Geometry: final body of the model. Coordinates: model frame, mm. A direction names the side the tool comes from. Give positions to 0.01 mm unless a question says otherwise; leave off trailing zeros. Order: outer loops, then holes, each group sorted by start corner. A loop starts at its lowest first (then second) coordinate and runs counter-clockwise, first axis right, second up. Notation, with made-up numbers: (-1.75, 65) -> (4.25, 65) arc R17 cw to (4.25, 96) -> close; hole circle Ø7 at (64.25, -30). An arc over 180 degrees is marked (long way). One line per question, with ' | ' between items. Start each with the question number.
(1) Section D-D (z = 27). Return loops of the section in (x, y), then the cut area to 3 significant figures.
(2) Section C-C (x = -8). Return loops of the section in (y, z), then the cut area to 3 significant figures.
(3) Set-up query: faces 1 (the face through (-18, 0, 9)), 2 (the face through (-44.45, -5, 6)), 3 (the face through (-33, -11.014, 6)), 4 (the face through (-6, -25.59, 29)), 5 (the face through (-21, -16, 12.7)). Return all of +Z, -Z, +X, -X, +Y, -Y with unobstructed straight access to the full face (end or side cutting, diameter ignored); none if empty.
(4) Ray query, L1, parallel to Y at x = -36.5, z = 4; L2, parallel to X at y = -6, z = 25; L3, parallel to Z at x = -19.5, y = -11.5. Return the intervals inside material, ascending.
(5) Mould query, pull axis Y, two halves, no side actions, for faces 6 (the face through (-18, -16, 0)), 7 (the face through (-18, -31.75, 9)), 8 (the face through (-6, -5.669, 29)). Classes: +Y half, -Y half, draft (parallel to the pull), parting line (faces both ways), or undercut.
(6) Section A-A (z = 2.5). Return loops of the section in (x, y).
(7) First-contact query: pin 1 Ø1.7 at (x, z) = (-8, 27.5) entering from +Y; pin 2 Ø4 at (x, y) = (-6, -14.5) entering from +Z; pin 3 Ø4.5 at (y, z) = (-16, 7) entering from -X; pin 4 Ø3 at (y, z) = (-20, 21) entering from -X. Flat tips, straight axial feed; report the tip coordinate or a pass-through.
(8) Section B-B (x = -41). Return loops of the section in (y, z).
```python
from build123d import *

# Parameters (mm, degrees)
F1_DEPTH = 31.75
F2_W     = 22.5849208206
F2_H     = 8.5840681568
F3_DEPTH = 1320.8
F5_DEPTH = 127


with BuildPart() as f1:
    # F0 (on Front) → F1 (new body)
    with BuildSketch(Plane.XZ):
        Polygon((-44.45, 0), (0, 0), (0, 31.75), (-12.7, 31.75), (-12.7, 12.7), (-44.45, 12.7), align=None)
    extrude(amount=F1_DEPTH)

    # F2 (on face) → F3 (cut)
    with BuildSketch(Plane.XY.offset(12.7)):
        with Locations((-33.1575395897, -15.3055558912)):
            Rectangle(F2_W, F2_H)
    extrude(amount=-F3_DEPTH, mode=Mode.SUBTRACT)

    # F4 (on Right) → F5 (cut)
    with BuildSketch(Plane.YZ):
        Polygon((-5.6687253527, 31.9069586694), (-25.590242818, 31.7449867725), (-25.590242818, 26.2379515916), (-5.6687253527, 26.2379515916), align=None)
    extrude(amount=-F5_DEPTH, mode=Mode.SUBTRACT)


solid = f1.part
```
Response:
1) outline: (-12.7, -31.75) -> (0, -31.75) -> (0, -25.59) -> (-12.7, -25.59) -> close; (-12.7, -5.67) -> (0, -5.67) -> (0, 0) -> (-12.7, 0) -> close | area: 150 mm^2
2) outline: (-31.75, 0) -> (0, 0) -> (0, 31.75) -> (-5.67, 31.75) -> (-5.67, 26.24) -> (-25.59, 26.24) -> (-25.59, 31.74) -> (-24.97, 31.75) -> (-31.75, 31.75) -> close | area: 898 mm^2
3) face 1: +Z, -Z, +X, -X, +Y | face 2: +Z, -Z, -X, +Y, -Y | face 3: +Z, -Z, -X | face 4: +X, -X | face 5: +Z, -X, +Y, -Y
4) L1: y = -31.75 to -19.6, -11.01 to 0 | L2: x = -12.7 to 0 | L3: z = 0 to 12.7
5) face 6: draft | face 7: -Y half | face 8: undercut
6) outline: (-44.45, -31.75) -> (0, -31.75) -> (0, 0) -> (-44.45, 0) -> (-44.45, -11.01) -> (-21.87, -11.01) -> (-21.87, -19.6) -> (-44.45, -19.6) -> close
7) pin 1: stops at y = 0 | pin 2: stops at z = 26.24 | pin 3: stops at x = -21.87 | pin 4: stops at x = -12.7
8) outline: (-31.75, 0) -> (-19.6, 0) -> (-19.6, 12.7) -> (-31.75, 12.7) -> close; (-11.01, 0) -> (0, 0) -> (0, 12.7) -> (-11.01, 12.7) -> close
